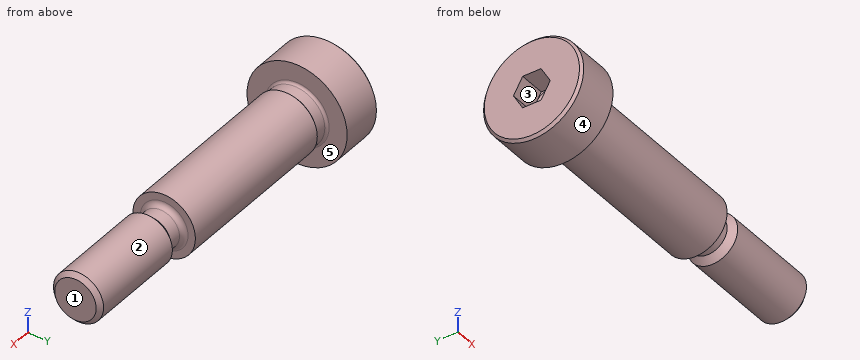
from build123d import *

# Parameters (mm, degrees)
CHAMFER1_SIZE = 0.4
HEX_2_DEPTH   = 4.2


# Read off the part's stored shape, not the designer's step: ThreadSchematic
with BuildPart() as part:
    # ThreadSchematic outline → ThreadSchematic (revolve)
    with BuildSketch(Plane.YX):
        with BuildLine():
            Line((0, 57), (0, 0))
            Line((0, 0), (8, 0))
            Line((8, 0), (8, 7))
            Line((8, 7), (5.11, 7))
            ThreePointArc((5.11, 7), (4.827157288, 7.117157288), (4.71, 7.4))
            Line((4.71, 7.4), (4.71, 9.2165))
            Line((4.71, 9.2165), (4.9935, 9.5))
            Line((4.9935, 9.5), (4.9935, 37))
            Line((4.9935, 37), (3.815, 37))
            ThreePointArc((3.815, 37), (3.249314575, 37.234314575), (3.015, 37.8))
            Line((3.015, 37.8), (3.015, 39.8))
            Line((3.015, 39.8), (4, 40.785))
            Line((4, 40.785), (4, 56.3095))
            Line((4, 56.3095), (3.3095, 57))
            Line((3.3095, 57), (0, 57))
        make_face()
    revolve(axis=Axis((0, 0, 0), (1, 0, 0)))

    # Chamfer1
    chamfer1_edges = [part.edges().sort_by_distance(p)[0] for p in [
        (0, -8, 0),
    ]]
    chamfer(chamfer1_edges, length=CHAMFER1_SIZE)

    # Sketch2 → PreBroach (revolve, cut)
    with BuildSketch(Plane.XY, mode=Mode.PRIVATE) as prebroach_sk:
        Polygon((0, 2.5475), (4.2, 2.5475), (5.670799811, 0), (0, 0), align=None)
    revolve(prebroach_sk.sketch.rotate(Axis((0, 0, 0), (1, 0, 0)), 90), axis=Axis((0, 0, 0), (1, 0, 0)), mode=Mode.SUBTRACT)

    # Sketch3 → Hex 2 (cut)
    with BuildSketch(Plane.ZY):
        Polygon((-2.5475, -1.470799811), (-2.5475, 1.470799811), (0, 2.941599622), (2.5475, 1.470799811), (2.5475, -1.470799811), (0, -2.941599622), align=None)
    extrude(amount=-HEX_2_DEPTH, mode=Mode.SUBTRACT)


solid = part.part
Design review of the part built by this model. Coordinates are the model's own, in mm. Face numbers are marked on the shaded views. A direction names the side the tool comes from. Round coordinates to 2 decimals unless told otherwise and drop trailing zeros. Loops run counter-clockwise (first coordinate to the right, second up) from the corner with the lowest first, then second, coordinate; pieces in that order, holes last. Notation, with made-up numbers: (-33.5, 89) -> (-3.5, 89) arc R30 cw to (-3.5, 123) -> close; hole circle Ø9 at (3, -17.5). An arc over 180 degrees is marked (long way). Use one line per item in the form item = value. Start each with the question number.
Q1. We need section B-B on x = 27.5. Give the boundary of the cut face in (y, z).
Q2. We need section A-A on x = 41.5. Give the boundary of the cut face in (y, z), then the cut area to 3 significant figures.
Q3. For pin 1 Ø2.5 at (x, y) = (1.5, 0.5) entering from -Z; pin 2 Ø2 at (x, z) = (49, -1) entering from -Y; pin 3 Ø5 at (x, z) = (46, 5.5) entering from -Y; pin 4 Ø5 at (x, y) = (14.5, 3.5) entering from +Z, all flat-tipped, find the tip position at first contact; note any pin that passes through.
Q4. Wall thickness on line 1 along X through (y, z) = (4.75, 3.5); line 2 along Z through (x, y) = (36, -0.25); line 3 along X through (y, z) = (-0.75, -3): over which ranges is each line inside the solid? List them lowest first. Write a range as [from, to].
Q5. Draft analysis for pull direction Y (two halves, no side actions). For the marked faces 3, 4 and 5, state which applies: +Y half, -Y half, draft (parallel to the pull), parting line (faces both ways), or undercut.
Q6. Machinability: for the marked faces 1 and 2, which of the approach directions +Z, -Z, +X, -X, +Y, -Y give a long, thin tool a straight path to every point of the face, cutting with its end or side? Answer none if there is none.
Calculated:
q1.outline = circle Ø9.99 at (0, 0)
q2.outline = circle Ø8 at (0, 0)
q2.area = 50.3 mm²
q3.pin_1 = -8
q3.pin_2 = -4
q3.pin_3 = -2.65
q3.pin_4 = 4.89
q4.line_1 = [0, 7]
q4.line_2 = [-4.99, 4.99]
q4.line_3 = [0, 37.46], [39.88, 57]
q5.face_3 = undercut
q5.face_4 = parting line
q5.face_5 = draft
q6.face_1 = +Z, -Z, +X, +Y, -Y
q6.face_2 = +X
